Here's how the part is built. I have some questions about the finished solid (model axes, mm). A direction names the side the tool comes from. Round coordinates to 2 decimals unless told otherwise and drop trailing zeros. Write each loop counter-clockwise with the first axis right and the second up, starting at its lowest first coordinate (ties: lowest second). Pieces come first, ordered by that corner, then holes. Notation, with made-up numbers: (81.5, 61.5) -> (92.5, 61.5) arc R20 cw to (92.5, 90.5) -> close; hole circle Ø2 at (82, 39.25). An arc over 180 degrees is marked (long way). Answer as CSV lines item,"result".
```python
from build123d import *
from build123d.topology import SkipClean

# Parameters (mm, degrees)
BOSS_EXTRUDE1_DEPTH = 2
BOSS_EXTRUDE2_START = 5
BOSS_EXTRUDE2_DEPTH = 5
BOSS_EXTRUDE3_START = 2
SKETCH3_R           = 3
SKETCH3_R_2         = 1.7
BOSS_EXTRUDE3_DEPTH = 2
SKETCH4_R           = 2.2
SKETCH4_R_2         = 1.7
BOSS_EXTRUDE4_DEPTH = 0.5
CHAMFER1_SIZE       = 0.5
FILLET1_R           = 0.5


with BuildPart() as part:
    # Sketch1 → Boss-Extrude1 (new body)
    with BuildSketch(Plane.XY):
        with BuildLine():
            Line((4.594082841, 4.876925553), (5.159993549, 5.442836262))
            ThreePointArc((5.159993549, 5.442836262), (0, 7.5), (-5.159993549, 5.442836262))
            Line((-5.159993549, 5.442836262), (-4.594082841, 4.876925553))
            ThreePointArc((-4.594082841, 4.876925553), (0, 6.7), (4.594082841, 4.876925553))
        make_face()
    extrude(amount=-BOSS_EXTRUDE1_DEPTH)

    # Sketch1<3> → Boss-Extrude2 (add)
    with BuildSketch(Plane.XY.offset(BOSS_EXTRUDE2_START)):
        with BuildLine():
            Line((4.594082841, 4.876925553), (5.159993549, 5.442836262))
            ThreePointArc((5.159993549, 5.442836262), (0, 7.5), (-5.159993549, 5.442836262))
            Line((-5.159993549, 5.442836262), (-4.594082841, 4.876925553))
            ThreePointArc((-4.594082841, 4.876925553), (0, 6.7), (4.594082841, 4.876925553))
        make_face()
    extrude(amount=-BOSS_EXTRUDE2_DEPTH)

    # Sketch3 → Boss-Extrude3 (add)
    # profile 1 of 3: a face of its own
    with BuildSketch(Plane.XY.offset(5).offset(BOSS_EXTRUDE3_START)):
        with BuildLine():
            Line((-4.594082841, 4.876925553), (-5.159993549, 5.442836262))
            Line((-5.159993549, 5.442836262), (-2.820975701, -1.02083108))
            ThreePointArc((-2.820975701, -1.02083108), (-2.892694114, 0.795185994), (-1.902774006, 2.31936437))
            Line((-1.902774006, 2.31936437), (-2.780654635, 4.745309242))
            ThreePointArc((-2.780654635, 4.745309242), (0, 5.5), (2.780654635, 4.745309242))
            Line((2.780654635, 4.745309242), (1.902774006, 2.31936437))
            ThreePointArc((1.902774006, 2.31936437), (2.711855639, 1.282902565), (3, 0))
            ThreePointArc((3, 0), (2.954904999, -0.518205025), (2.820975701, -1.02083108))
            Line((2.820975701, -1.02083108), (5.159993549, 5.442836262))
            Line((5.159993549, 5.442836262), (4.594082841, 4.876925553))
            ThreePointArc((4.594082841, 4.876925553), (0, 6.7), (-4.594082841, 4.876925553))
        make_face()
    # profile 2 of 3: a face of its own
    with BuildSketch(Plane.XY.offset(5).offset(BOSS_EXTRUDE3_START)):
        with BuildLine():
            Line((-5.159993549, 5.442836262), (-4.594082841, 4.876925553))
            ThreePointArc((-4.594082841, 4.876925553), (0, 6.7), (4.594082841, 4.876925553))
            Line((4.594082841, 4.876925553), (5.159993549, 5.442836262))
            ThreePointArc((5.159993549, 5.442836262), (0, 7.5), (-5.159993549, 5.442836262))
        make_face()
    # profile 3 of 3: a face of its own
    with BuildSketch(Plane.XY.offset(5).offset(BOSS_EXTRUDE3_START)):
        Circle(SKETCH3_R)
        Circle(SKETCH3_R_2, mode=Mode.SUBTRACT)
    extrude(amount=-BOSS_EXTRUDE3_DEPTH)

    # Sketch4 → Boss-Extrude4 (add)
    with SkipClean():  # the faces are left unmerged after this step: merging them gives an invalid solid
        with BuildSketch(Plane(origin=(0, 0, 5), x_dir=(-1, 0, 0), z_dir=(0, 0, -1))):
            with Locations(Location((0, 0, 0), (0, 0, 180))):
                Circle(SKETCH4_R)
            Circle(SKETCH4_R_2, mode=Mode.SUBTRACT)
        extrude(amount=BOSS_EXTRUDE4_DEPTH)
    add(part.part.scale(1), mode=Mode.REPLACE)  # the faces are merged on a copy

    # Chamfer1
    chamfer1_edges = [part.edges().sort_by_distance(p)[0] for p in [
        (-2.2, 0, 5),
    ]]
    chamfer(chamfer1_edges, length=CHAMFER1_SIZE - 0.0001)  # a hair under: the kernel refuses the full size

    # Fillet1
    fillet1_edges = [part.edges().sort_by_distance(p)[0] for p in [
        (2.780654635, 4.745309242, 6),
        (1.902774006, 2.31936437, 6),
        (-1.902774006, 2.31936437, 6),
        (-2.780654635, 4.745309242, 6),
    ]]
    fillet(fillet1_edges, radius=FILLET1_R)


solid = part.part
```
1. On a 3-axis mill with a long thin cutter (end or side, diameter ignored), from which of +Z, -Z, +X, -X, +Y, -Y can I reach the whole of each face in a straight line? I mean faces 5 (the face through (-1.9, 2.2, 5)), 6 (the face through (2.38, 3.64, 6.01)), 7 (the face through (-4.01, 2.26, 6.01)). Say none if no direction works.
Numbers:
face 5,"-Z"
face 6,"+Z, -Z"
face 7,"+Z, -Z, -X, -Y"
2. For pin 1 Ø1 at (x, z) = (-4, 0.5) entering from -Y; pin 2 Ø1.5 at (x, z) = (-4, 1) entering from +Y; pin 3 Ø5 at (x, y) = (0.5, 0) entering from -Z; pin 4 Ø2 at (x, y) = (4, 0.5) entering from +Z, each with a flat end and sliding along its axis, tell me the tip position at first contact or that it passes through.
Numbers:
pin 1,"stops at y = 4.96"
pin 2,"stops at y = 6.76"
pin 3,"stops at z = 4.5"
pin 4,"stops at z = 7"
3. If we mould it in two halves opening along Y, with no side actions, what happens to faces 1 (the face through (0, 3, 6)), 2 (the face through (0.1, 7.5, 2.6)), 3 (the face through (-2.373, 3.617, 6.014)), 4 (the face through (-2, 0, 4.5))? For each: released by +Y, released by -Y, zero draft, split by the parting line, or undercut.
Numbers:
face 1,"undercut"
face 2,"released by +Y"
face 3,"undercut"
face 4,"zero draft"
4. If I drill on line 1 (X direction, y = 1.5, z = 6.25); line 2 (Y direction, x = 0, z = 4.85); line 3 (X direction, y = 0.25, z = 6.25), over which ranges is the centre line in solid material (lowest first)?
Numbers:
line 1,"x = -3.73 to -0.8, 0.8 to 3.73"
line 2,"y = -2.55 to -1.7, 1.7 to 2.55, 6.7 to 7.5"
line 3,"x = -3.28 to -1.68, 1.68 to 3.28"
5. Suppose I cut it at B-B on z = 6. Please give me the cut outline in (x, y).
Numbers:
outline,"(-5.16, 5.44) -> (-2.82, -1.02) arc R3 ccw to (2.82, -1.02) -> (5.16, 5.44) arc R7.5 ccw to start; hole (-2.63, 4.34) -> (-2.12, 2.92) arc R0.5 ccw to (-1.41, 2.65) arc R3 cw to (1.41, 2.65) arc R0.5 ccw to (2.12, 2.92) -> (2.63, 4.34) arc R0.5 ccw to (2.38, 4.96) arc R5.5 ccw to (-2.38, 4.96) arc R0.5 ccw to start; hole circle Ø3.4 at (0, 0)"
6. Suppose I cut it at A-A on x = 0. Count the separate pieces of the cut face and the enclosed holes in it, and give its area (3 significant figures).
Numbers:
separate pieces,"3"
enclosed holes,"0"
area,"15.5 mm^2"
7. Suppose I cut it at D-D on y = 3.25. Please give me the cut outline in (x, z).
Numbers:
outline,"(-4.37, 5) -> (-2.24, 5) -> (-2.24, 7) -> (-4.37, 7) -> close; (2.24, 5) -> (4.37, 5) -> (4.37, 7) -> (2.24, 7) -> close"
